Model file for the job. Use its own axes, mm. A direction names the side the tool comes from. Round coordinates to 2 decimals unless told otherwise and drop trailing zeros. Order: outer loops, then holes, each group sorted by start corner. A loop starts at its lowest first (then second) coordinate and runs counter-clockwise, first axis right, second up. Notation, with made-up numbers: (38.5, -23.75) -> (51.5, -23.75) arc R23 ccw to (51.5, -7.75) -> close; hole circle Ø3 at (14, -3.75). An arc over 180 degrees is marked (long way). Put each result on its own line as item: value. Start each with the question number.
Q1. Cut at C-C, the plane y = -6.25. List the corners of the cut face in (x, z).
Q2. Pull direction Z, two halves, no side cores. Call faces 4 (the face through (0, 0, 1)), 5 (the face through (-6, 0, 2)), 6 (the face through (3, -3, 5)): released by +Z, released by -Z, zero draft, split by the parting line, or undercut.
Q3. Cut at A-A, the plane y = 0. List the corners of the cut face in (x, z).
Q4. Cut at B-B, the plane z = 8. List the corners of the cut face in (x, y).
Q5. 3-axis set-ups, long thin cutter, end or side, ignore diameter. For faces 1 (the face through (-0.867, 3.905, 0.493)), 2 (the face through (2, 6, 1)), 3 (the face through (-0.867, -3.905, 6.972)): which of +Z, -Z, +X, -X, +Y, -Y reach the whole face in a straight line?
Q6. Flat gauge pins, fed straight in: P1, Ø2.5, axis at x = 0.5, y = -1.5, coming from the -Z side; P2, Ø4, axis at y = -1, z = 5, coming from the +X side; P3, Ø4, axis at x = 6, z = 6, coming from the -Y side. Where does each tip first touch, or does it go through?
Q7. Probe L1, parallel to Z at x = 2, y = -7; L2, parallel to Y at x = 0, z = 0.25; L3, parallel to Y at x = 0, z = 7.85. List the from-to ranges inside material, lowest first.
from build123d import *

# Parameters (mm, degrees)
F0_R      = 7.5
F1_DEPTH  = 1
F2_R      = 6
F3_DEPTH  = 3
F4_R      = 7.5
F4_R_2    = 6
F5_DEPTH  = 1
F7_R      = 4
F8_DEPTH  = 4
F9_R      = 2.5
F10_DEPTH = 2
F11_R     = 4
F12_DEPTH = 1


with BuildPart() as f1:
    # F0 (on Top) → F1 (new body)
    with BuildSketch(Plane.XY):
        Circle(F0_R)
    extrude(amount=F1_DEPTH)

    # F2 (on face) → F3 (join)
    with BuildSketch(Plane.XY.offset(1)):
        Circle(F2_R)
    extrude(amount=F3_DEPTH)

    # F4 (on face) → F5 (join)
    with BuildSketch(Plane.XY.offset(4)):
        Circle(F4_R)
        Circle(F4_R_2, mode=Mode.SUBTRACT)
        Circle(F4_R_2)
    extrude(amount=F5_DEPTH)

    # F7 (on face) → F8 (join)
    with BuildSketch(Plane.XY.offset(5)):
        Circle(F7_R)
    extrude(amount=F8_DEPTH)

    # F9 (on face) → F10 (cut)
    with BuildSketch(Plane.XY.offset(9)):
        Circle(F9_R)
    extrude(amount=-F10_DEPTH, mode=Mode.SUBTRACT)

    # F11 (on face) → F12 (cut)
    with BuildSketch(Plane(origin=(0, 0, 0), x_dir=(1, 0, 0), z_dir=(0, 0, -1))):
        Circle(F11_R)
    extrude(amount=-F12_DEPTH, mode=Mode.SUBTRACT)


solid = f1.part
Ans:
1. outline: (-4.15, 0) -> (4.15, 0) -> (4.15, 1) -> (-4.15, 1) -> close; (-4.15, 4) -> (4.15, 4) -> (4.15, 5) -> (-4.15, 5) -> close
2. face 4: released by -Z
2. face 5: undercut
2. face 6: released by +Z
3. outline: (-7.5, 0) -> (-4, 0) -> (-4, 1) -> (4, 1) -> (4, 0) -> (7.5, 0) -> (7.5, 1) -> (6, 1) -> (6, 4) -> (7.5, 4) -> (7.5, 5) -> (4, 5) -> (4, 9) -> (2.5, 9) -> (2.5, 7) -> (-2.5, 7) -> (-2.5, 9) -> (-4, 9) -> (-4, 5) -> (-7.5, 5) -> (-7.5, 4) -> (-6, 4) -> (-6, 1) -> (-7.5, 1) -> close
4. outline: circle Ø8 at (0, 0); hole circle Ø5 at (0, 0)
5. face 1: -Z
5. face 2: none
5. face 3: +Z
6. P1: stops at z = 1
6. P2: stops at x = 7.5
6. P3: stops at y = -6.17
7. L1: z = 0 to 1, 4 to 5
7. L2: y = -7.5 to -4, 4 to 7.5
7. L3: y = -4 to -2.5, 2.5 to 4
